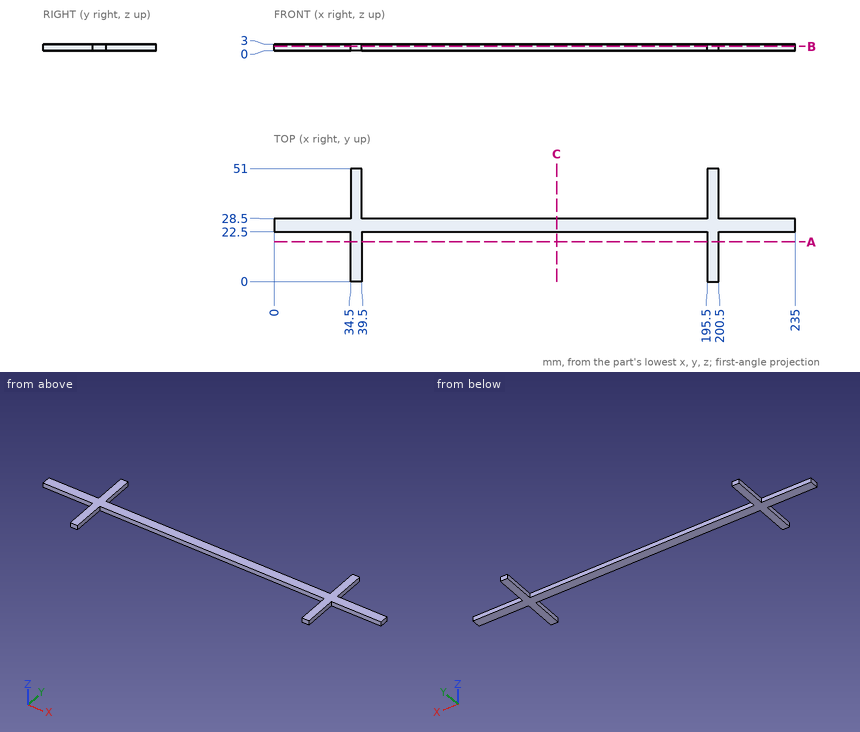
Drawing for the job (mm, zero at the part's lowest x, y, z). Give positions to 0.01 mm unless a question says otherwise; leave off trailing zeros. Loops run counter-clockwise (first coordinate to the right, second up) from the corner with the lowest first, then second, coordinate; pieces in that order, holes last.
Item 1: Drop flat-ended pins along their axis: P1, Ø1.5, axis at x = 49, z = 1, coming from the -Y side; P2, Ø1, axis at x = 163, z = 1, coming from the +Y side; P3, Ø1.5, axis at y = 9, z = 2.5, coming from the -X side. Give the stop position or say it passes through.
Check values:
P1: stops at y = 22.5
P2: stops at y = 28.5
P3: stops at x = 34.5
Item 2: Slice it at B-B (z = 1.9). Write the cut outline in (x, y), plus the area to 3 significant figures.
Check values:
outline: (0, 22.5) - (34.5, 22.5) - (34.5, 0) - (39.5, 0) - (39.5, 22.5) - (195.5, 22.5) - (195.5, 0) - (200.5, 0) - (200.5, 22.5) - (235, 22.5) - (235, 28.5) - (200.5, 28.5) - (200.5, 51) - (195.5, 51) - (195.5, 28.5) - (39.5, 28.5) - (39.5, 51) - (34.5, 51) - (34.5, 28.5) - (0, 28.5) - close
area: 1,860 mm2
Item 3: Slice it at C-C (x = 127.5). Write the cut outline in (y, z), plus the area to 3 significant figures.
Check values:
outline: (22.5, 0) - (28.5, 0) - (28.5, 3) - (22.5, 3) - close
area: 18.0 mm2
Item 4: Drill centre lines: line 1 along X through (y, z) = (44.5, 2.7); line 2 along Y through (x, z) = (122, 2.4). Where is each one in solid material? Low to high.
Check values:
line 1: x = 34.5 to 39.5, 195.5 to 200.5
line 2: y = 22.5 to 28.5
Item 5: Slice it at A-A (y = 18). Write the cut outline in (x, z), plus the area to 3 significant figures.
Check values:
outline: (34.5, 0) - (39.5, 0) - (39.5, 3) - (34.5, 3) - close; (195.5, 0) - (200.5, 0) - (200.5, 3) - (195.5, 3) - close
area: 30.0 mm2
